```python
from build123d import *

# Parameters (mm, degrees)
F1_DEPTH = 20
F2_R     = 2.5
F3_DEPTH = 20
F4_R     = 2.5
F5_DEPTH = 20


with BuildPart() as f1:
    # F0 (on Top) → F1 (new body)
    with BuildSketch(Plane.XY):
        with BuildLine():
            Line((49, -19), (49, 19))
            Line((49, 19), (-49, 19))
            Line((-49, 19), (-49, -19))
            Line((-49, -19), (-23.25, -19))
            ThreePointArc((-23.25, -19), (0, 4.25), (23.25, -19))
            Line((23.25, -19), (49, -19))
        make_face()
    extrude(amount=F1_DEPTH)

    # F2 (on face) → F3 (cut)
    with BuildSketch(Plane(origin=(0, 19, 0), x_dir=(-1, 0, 0), z_dir=(0, 1, 0))):
        with Locations((-37, 10)):
            Circle(F2_R)
        with Locations((37, 10)):
            Circle(F2_R)
    extrude(amount=-F3_DEPTH, mode=Mode.SUBTRACT)

    # F4 (on face) → F5 (cut)
    with BuildSketch(Plane.XY.offset(20)):
        with Locations((34, -7)):
            Circle(F4_R)
    extrude(amount=-F5_DEPTH, mode=Mode.SUBTRACT)


solid = f1.part
```
The model under review builds one solid part; all positions refer to its coordinate system, in mm. A direction names the side the tool comes from. Round coordinates to 2 decimals unless told otherwise and drop trailing zeros. Loops run counter-clockwise (first coordinate to the right, second up) from the corner with the lowest first, then second, coordinate; pieces in that order, holes last. Notation, with made-up numbers: M 44,-33 L 69,-33 A28 cw 69,-10 Z; hole C 11.25,15.25 d6. An arc over 180 degrees is marked long. Answer as a JSON object with one key per item and string values.
(1) Take a section at C-C on x = -37. Give the boundary of the cut face in (y, z), and give its area (3 significant figures).
Resolved:
{"outline": "M -19,0 L 19,0 L 19,7.5 L -1,7.5 L -1,12.5 L 19,12.5 L 19,20 L -19,20 Z", "area": "660 mm²"}
(2) Draft analysis for pull direction Z (two halves, no side actions). For faces 1 (the flat face through (-37, -1, 10)), 2 (the flat face through (-0.7, 4.5, 20)), 3 (the flat face through (49, 0, 10)), state which applies: released by +Z, released by -Z, zero draft, split by the parting line, or undercut.
Resolved:
{"face 1": "undercut", "face 2": "released by +Z", "face 3": "zero draft"}
(3) To check wall thickness, follow line 1 along Z through (x, y) = (-37, 12); line 2 along X through (y, z) = (13, 12); line 3 along Y through (x, z) = (34, 4.75). State the ranges of each line that lie inside material, in increasing order.
Resolved:
{"line 1": "0 to 7.5, 12.5 to 20", "line 2": "-49 to -38.5, -35.5 to 35.5, 38.5 to 49", "line 3": "-19 to -9.5, -4.5 to 19"}
(4) Clearance check with flat-ended pins moving along their axes: P1, Ø3, axis at x = -37, z = 10, coming from the +Y side; P2, Ø3, axis at x = 34, y = -7, coming from the -Z side; P3, Ø1.5, axis at x = 18, z = 13.5, coming from the -Y side. State where each tip first meets the part, or that it passes through.
Resolved:
{"P1": "y = -1", "P2": "through", "P3": "y = -5.25"}
(5) Tool access review of faces 4 (the cylindrical face through (36.31, -7.96, 10.14)), 5 (the cylindrical face through (-39.31, 9.14, 9.04)): name each direction out of +Z, -Z, +X, -X, +Y, -Y from which nothing blocks a thin tool from reaching the whole face with its end or side.
Resolved:
{"face 4": "+Z, -Z", "face 5": "+Y"}
(6) Take a section at B-B on y = -16. Give the boundary of the cut face in (x, z), and give its area (3 significant figures).
Resolved:
{"outline": "M -49,0 L -23.06,0 L -23.06,20 L -49,20 Z; M 23.06,0 L 49,0 L 49,20 L 23.06,20 Z", "area": "1,040 mm²"}
(7) Take a section at D-D on y = -7. Give the boundary of the cut face in (x, z), and give its area (3 significant figures).
Resolved:
{"outline": "M -49,0 L -19.91,0 L -19.91,20 L -49,20 Z; M 19.91,0 L 31.5,0 L 31.5,20 L 19.91,20 Z; M 36.5,0 L 49,0 L 49,20 L 36.5,20 Z", "area": "1,060 mm²"}
(8) Take a section at A-A on z = 4. Give the boundary of the cut face in (x, y), and give its area (3 significant figures).
Resolved:
{"outline": "M -49,-19 L -23.25,-19 A23.25 cw 23.25,-19 L 49,-19 L 49,19 L -49,19 Z; hole C 34,-7 d5", "area": "2,860 mm²"}
